Could you check a few things on this model? Use its own coordinates, in mm. Face numbers are marked on the shaded views. A direction names the side the tool comes from. Round coordinates to 2 decimals unless told otherwise and drop trailing zeros. Write each loop counter-clockwise with the first axis right and the second up, starting at its lowest first coordinate (ties: lowest second). Pieces come first, ordered by that corner, then holes. Notation, with made-up numbers: (-33.75, 8.25) -> (-4.75, 8.25) arc R15 ccw to (-4.75, 17.25) -> close; hole circle Ø4 at (39.5, 46.5). An arc over 180 degrees is marked (long way). One line per question, with ' | ' between items. Start each with the question number.
1. If I drill on line 1 along Z through (x, y) = (17.5, 44); line 2 along Y through (x, z) = (62, -16.75); line 3 along X through (y, z) = (133, -14), over which ranges is the centre line in solid material (lowest first)? Write a range as [from, to].
2. Imagine slicing it at A-A, the plane x = 25.5. List the corners of the cut face in (y, z) for me.
3. For the marked faces 1 and 2, which set-ups out of +Z, -Z, +X, -X, +Y, -Y let a thin tool reach every point of the face, with its end or its side?
4. Imagine slicing it at B-B, the plane y = 15. List the corners of the cut face in (x, z) for me.
5. Imagine slicing it at C-C, the plane z = -16.5. List the corners of the cut face in (x, y) for me, and give its area (3 significant figures).
6. For pin 1 Ø2 at (x, z) = (125, -1.5) entering from +Y; pin 2 Ø1.2 at (y, z) = (151.5, -2) entering from +X; pin 3 Ø1.5 at (x, z) = (150, -4.5) entering from +Y, each with a flat end and sliding along its axis, tell me the tip position at first contact or that it passes through.
from build123d import *

# Parameters (mm, degrees)
PAD_DEPTH     = 2
SKETCH001_W   = 5
SKETCH001_H   = 25
PAD001_DEPTH  = 220
SKETCH002_W   = 5
SKETCH002_H   = 25
PAD002_DEPTH  = 220
FILLET_R      = 3
FILLET001_R   = 3
CHAMFER_ANGLE = 5
CHAMFER_SIZE  = 21


with BuildPart() as part:
    # Sketch → Pad (new body)
    with BuildSketch(Plane.XY):
        with BuildLine():
            Line((0, 0), (0, 220))
            ThreePointArc((40.642952, 189.925797), (25.279968, 211.663917), (0, 220))
            Line((40.642952, 189.925797), (68.840599, 93.983665))
            ThreePointArc((68.840599, 93.983665), (78.011612, 77.552663), (93.378142, 66.69195))
            Line((189.925797, 40.642952), (93.378142, 66.69195))
            ThreePointArc((220, 0), (211.663917, 25.279968), (189.925797, 40.642952))
            Line((220, 0), (0, 0))
        make_face()
    extrude(amount=PAD_DEPTH)

    # Sketch001 → Pad001 (join)
    with BuildSketch(Plane.YZ):
        with Locations((2.5, -12.5)):
            Rectangle(SKETCH001_W, SKETCH001_H)
    extrude(amount=PAD001_DEPTH)

    # Sketch002 → Pad002 (join)
    with BuildSketch(Plane.XZ):
        with Locations((2.5, -12.5)):
            Rectangle(SKETCH002_W, SKETCH002_H)
    extrude(amount=-PAD002_DEPTH)

    # Fillet
    fillet_edges = [part.edges().sort_by_distance(p)[0] for p in [
        (112.352429, 5, 0),
    ]]
    fillet(fillet_edges, radius=FILLET_R)

    # Fillet001
    fillet001_edges = [part.edges().sort_by_distance(p)[0] for p in [
        (5, 113.852429, 0),
        (5, 5, -14),
    ]]
    fillet(fillet001_edges, radius=FILLET001_R)

    # Chamfer
    chamfer_edges = [part.edges().sort_by_distance(p)[0] for p in [
        (114, 5, -25),
    ]]
    chamfer_side = part.faces().sort_by_distance((114.020092, 5, -13.997627))[0]
    chamfer(chamfer_edges, length=CHAMFER_SIZE, angle=CHAMFER_ANGLE, reference=chamfer_side)


solid = part.part
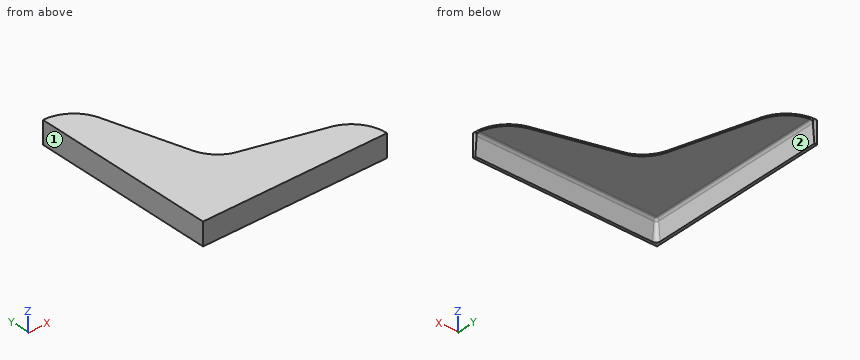
Geometry results:
1) line 1: z = [0, 2] | line 2: y = [0, 3.88] | line 3: x = [0, 4.13]
2) outline: (0, -25) -> (3.16, -25) -> (5, -4) -> (5, -3) arc R3 cw to (8, 0) -> (211.5, 0) -> (211.5, 2) -> (0, 2) -> close
3) face 1: +Z, -Z, -X, +Y, -Y | face 2: -Z, +X, +Y
4) outline: (0, -25) -> (3.16, -25) -> (5, -4) -> (5, -3) arc R3 cw to (8, 0) -> (217.26, 0) -> (217.26, 2) -> (0, 2) -> close
5) outline: (0, 0) -> (220, 0) -> (220, 3.91) -> (8, 3.91) arc R4.09 cw to (3.91, 8) -> (3.91, 220) -> (0, 220) -> close | area: 1,710 mm2
6) pin 1: stops at y = 6.34 | pin 2: stops at x = 5.46 | pin 3: stops at y = 5
